```python
from build123d import *

# Parameters (mm, degrees)
SKETCH2_R           = 30
SKETCH2_R_2         = 4
SKETCH2_R_3         = 1.75
BOSS_EXTRUDE1_DEPTH = 3
SKETCH3_R           = 8
SKETCH3_R_2         = 4
BOSS_EXTRUDE2_DEPTH = 10
SKETCH4_R           = 1.5
CUT_EXTRUDE2_DEPTH  = 4
SKETCH12_R          = 1.5
CUT_EXTRUDE3_DEPTH  = 11.49377522
CIRPATTERN1_COUNT   = 3


with BuildPart() as part:
    # Sketch2 → Boss-Extrude1 (new body)
    with BuildSketch(Plane.XY):
        Circle(SKETCH2_R)
        Circle(SKETCH2_R_2, mode=Mode.SUBTRACT)
        with Locations((0, -22)):
            Circle(SKETCH2_R_3, mode=Mode.SUBTRACT)
        with Locations((-19.052558883, 11)):
            Circle(SKETCH2_R_3, mode=Mode.SUBTRACT)
        with Locations((19.052558883, 11)):
            Circle(SKETCH2_R_3, mode=Mode.SUBTRACT)
    extrude(amount=BOSS_EXTRUDE1_DEPTH)

    # Sketch3 → Boss-Extrude2 (add)
    with BuildSketch(Plane.XY.offset(3)):
        Circle(SKETCH3_R)
        Circle(SKETCH3_R_2, mode=Mode.SUBTRACT)
    extrude(amount=BOSS_EXTRUDE2_DEPTH)

    # Sketch4 → Cut-Extrude2 (cut, through all)
    with BuildSketch(Plane.XY.offset(3)):
        with Locations((-6.5, 11.258330249)):
            Circle(SKETCH4_R)
        with Locations((13, 0)):
            Circle(SKETCH4_R)
        with Locations((-6.5, -11.258330249)):
            Circle(SKETCH4_R)
        with Locations((6.5, 11.258330249)):
            Circle(SKETCH4_R)
        with Locations((6.5, -11.258330249)):
            Circle(SKETCH4_R)
        with Locations((-13, 0)):
            Circle(SKETCH4_R)
    extrude(amount=-CUT_EXTRUDE2_DEPTH, mode=Mode.SUBTRACT)

    # Sketch12 → Cut-Extrude3 (cut)
    with BuildSketch(Plane(origin=(0, 0, 0), x_dir=(1, 0, 0), z_dir=(0, 1, 0))):
        with Locations((0, -8)):
            Circle(SKETCH12_R)
    cut_extrude3 = extrude(amount=-CUT_EXTRUDE3_DEPTH, mode=Mode.SUBTRACT)

    # CirPattern1: Cut-Extrude3 ×3 about axis
    cirpattern1_axis = Axis((0, 0, 0), (0, 0, -1))
    for i in range(1, CIRPATTERN1_COUNT):
        add(cut_extrude3.rotate(cirpattern1_axis, i * 360 / CIRPATTERN1_COUNT), mode=Mode.SUBTRACT)


solid = part.part
```
Work out the finished part from the listing and answer in its coordinate system (mm). A direction names the side the tool comes from. Coordinates: 2 decimals unless noted, no trailing zeros. Order: outer loops, then holes, each group sorted by start corner. A loop starts at its lowest first (then second) coordinate and runs counter-clockwise, first axis right, second up. Notation, with made-up numbers: (72.5, 49.25) - (105.5, 49.25) arc R19 cw to (105.5, 79.25) - close; hole circle Ø8 at (60.5, 44). An arc over 180 degrees is marked (long way). Answer as a JSON object with one key per item and string values.
1. Find section C-C on x = -13. Determine the outline of the cut face in (y, z).
Output values:
{"outline": "(-27.04, 0) - (-1.5, 0) - (-1.5, 3) - (-27.04, 3) - close; (1.5, 0) - (27.04, 0) - (27.04, 3) - (1.5, 3) - close"}
2. The mould has two halves that part along X. Classify faces 1 (the face through (6, 0, 0)), 2 (the face through (-29.97, 1.32, 1.48)), 3 (the face through (-7.69, 10.346, 1.521)): +X half, -X half, draft (parallel to the pull), parting line (faces both ways), or undercut.
Output values:
{"face 1": "draft", "face 2": "parting line", "face 3": "undercut"}
3. Each of these flat-tipped pins is pushed along its axis until it touches: P1, Ø6, axis at y = -0.5, z = 9, coming from the +X side; P2, Ø2.5, axis at x = 0, z = 8, coming from the -Y side; P3, Ø3, axis at y = 7, z = 10.5, coming from the -X side. Where does it stop, or does it pass through?
Output values:
{"P1": "stops at x = 8", "P2": "stops at y = 3.8", "P3": "stops at x = -5.81"}
4. Consider line 1 (Z direction, x = 2, y = -8.5); line 2 (Y direction, x = 19, z = 0.5); line 3 (Y direction, x = 13.5, z = 0.5). Determine where each line is inside the solid, lowest interval first.
Output values:
{"line 1": "z = 0 to 3", "line 2": "y = -23.22 to 9.25, 12.75 to 23.22", "line 3": "y = -26.79 to -1.41, 1.41 to 26.79"}
5. Find section D-D on z = 1. Count the separate pieces of the cut face and the enclosed holes in it, plus the area to 3 significant figures.
Output values:
{"separate pieces": "1", "enclosed holes": "10", "area": "2,710 mm²"}
6. Find section B-B on y = -22. Determine the outline of the cut face in (x, z).
Output values:
{"outline": "(-20.4, 0) - (-1.75, 0) - (-1.75, 3) - (-20.4, 3) - close; (1.75, 0) - (20.4, 0) - (20.4, 3) - (1.75, 3) - close"}
7. Find section A-A on x = 0. Determine the outline of the cut face in (y, z), plus the area to 4 significant figures.
Output values:
{"outline": "(-30, 0) - (-23.75, 0) - (-23.75, 3) - (-30, 3) - close; (-20.25, 0) - (-4, 0) - (-4, 6.5) - (-8, 6.5) - (-8, 3) - (-20.25, 3) - close; (-8, 9.5) - (-4, 9.5) - (-4, 13) - (-8, 13) - close; (4, 0) - (30, 0) - (30, 3) - (8, 3) - (8, 13) - (4, 13) - close", "area": "213.5 mm²"}
8. A tool of negligible diameter and unlimited length cuts with its end or side. For faces 4 (the face through (-0.867, -3.905, 6.409)), 5 (the face through (-1.5, -5.83, 7.93)), 6 (the face through (-1.73, -7.81, 7.93)), from which of +Z, -Z, +X, -X, +Y, -Y can it reach the whole face along a straight path? Write none if from no direction.
Output values:
{"face 4": "+Z, -Z", "face 5": "-Y", "face 6": "+Z"}
